from build123d import *

# Parameters (mm, degrees)
EXTRUDE_1_DEPTH     = 10
SKETCH_2_R          = 3
CUT_EXTRUDE_1_DEPTH = 10
LPATTERN1_COUNT     = 3
LPATTERN1_PITCH     = 50


with BuildPart() as part:
    # 草圖1 → 填料-伸長1 (new body)
    with BuildSketch(Plane.XY):
        Polygon((-40.155141061, 7.219614063), (-80.155141061, 7.219614063), (-80.155141061, 102.329702578), (-160.155141061, 102.329702578), (-160.155141061, 137.329702578), (39.844858939, 137.329702578), (39.844858939, 102.329702578), (-40.155141061, 102.329702578), align=None)
    extrude(amount=EXTRUDE_1_DEPTH)

    # 草圖2 → 除料-伸長1 (cut)
    with BuildSketch(Plane.XY.offset(10)):
        with Locations((-10.155141061, 117.189491535)):
            Circle(SKETCH_2_R)
    cut_extrude_1 = extrude(amount=-CUT_EXTRUDE_1_DEPTH, mode=Mode.SUBTRACT)

    # LPattern1: 除料-伸長1 ×3
    with Locations(*[(-i * LPATTERN1_PITCH, 0, 0) for i in range(1, LPATTERN1_COUNT)]):
        add(cut_extrude_1, mode=Mode.SUBTRACT)


solid = part.part
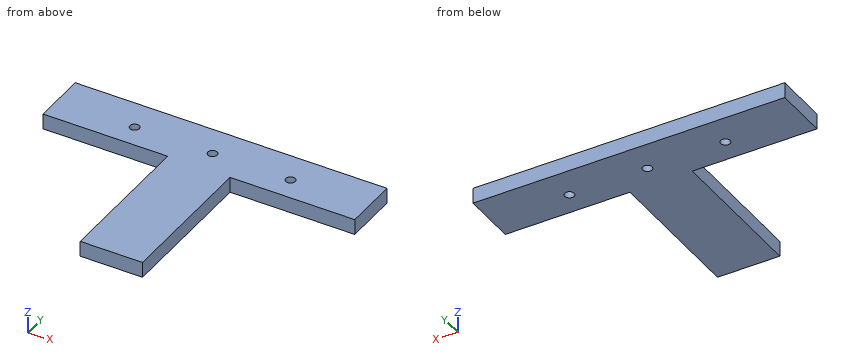
CAD build for the part. Positions are in the model's coordinates, mm. Give positions to 0.01 mm unless a question says otherwise; leave off trailing zeros. Write each loop counter-clockwise with the first axis right and the second up, starting at its lowest first coordinate (ties: lowest second). Pieces come first, ordered by that corner, then holes. Notation, with made-up numbers: M 66.25,45 L 95.25,45 A6 cw 95.25,53 Z; hole C -39.75,41 d10. An arc over 180 degrees is marked long. Put each result on its own line as item: value. Start each with the question number.
(1) Band-saw the part on A-A, the plane z = 8.25. Write the cut outline in (x, y), and give its area (3 significant figures).
(2) Flat gauge pins, fed straight in: pin 1 Ø1 at (y, z) = (93.5, 1.5) entering from +X; pin 2 Ø12 at (x, y) = (-86, 29.5) entering from -Z; pin 3 Ø3 at (x, z) = (-114, 6.5) entering from -Y; pin 4 Ø3 at (y, z) = (69, 7) entering from -X. Where does each tip first touch, or does it go through?
(3) Band-saw the part on B-B, the plane x = -118.5. Write the cut outline in (y, z).
(4) Band-saw the part on C-C, the plane y = 69. Write the cut outline in (x, z), and give its area (3 significant figures).
(5) Probe L1, parallel to Y at x = 3, z = 5.5; L2, parallel to Y at x = -60, z = 8; L3, parallel to X at y = 44, z = 5. List the from-to ranges inside material, lowest first.
Response values:
1. outline: M -160.16,102.33 L -80.16,102.33 L -80.16,7.22 L -40.16,7.22 L -40.16,102.33 L 39.84,102.33 L 39.84,137.33 L -160.16,137.33 Z; hole C -110.16,117.19 d6; hole C -60.16,117.19 d6; hole C -10.16,117.19 d6
1. area: 10,700 mm2
2. pin 1: stops at x = -40.16
2. pin 2: stops at z = 0
2. pin 3: stops at y = 102.33
2. pin 4: stops at x = -80.16
3. outline: M 102.33,0 L 137.33,0 L 137.33,10 L 102.33,10 Z
4. outline: M -80.16,0 L -40.16,0 L -40.16,10 L -80.16,10 Z
4. area: 400 mm2
5. L1: y = 102.33 to 137.33
5. L2: y = 7.22 to 114.19, 120.19 to 137.33
5. L3: x = -80.16 to -40.16
